from build123d import *

# Parameters (mm, degrees)
ESBO_O1_W                = 90
ESBO_O1_H                = 100
ESBO_O1_W_2              = 13
ESBO_O1_H_2              = 16
RESSALTO_EXTRUS_O1_DEPTH = 2
ESBO_O2_W                = 90
ESBO_O2_H                = 100
ESBO_O2_W_2              = 86
ESBO_O2_H_2              = 96
RESSALTO_EXTRUS_O2_DEPTH = 7


with BuildPart() as part:
    # Esboço1 → Ressalto-extrusão1 (new body)
    with BuildSketch(Plane.XY):
        Rectangle(ESBO_O1_W, ESBO_O1_H)
        with Locations((35.5, 37)):
            Rectangle(ESBO_O1_W_2, ESBO_O1_H_2, mode=Mode.SUBTRACT)
        with Locations((35.5, -37)):
            Rectangle(ESBO_O1_W_2, ESBO_O1_H_2, mode=Mode.SUBTRACT)
        with Locations((-35.5, -37)):
            Rectangle(ESBO_O1_W_2, ESBO_O1_H_2, mode=Mode.SUBTRACT)
        with Locations((-35.5, 37)):
            Rectangle(ESBO_O1_W_2, ESBO_O1_H_2, mode=Mode.SUBTRACT)
    extrude(amount=RESSALTO_EXTRUS_O1_DEPTH)

    # Esboço2 → Ressalto-extrusão2 (add)
    with BuildSketch(Plane.XY.offset(2)):
        Rectangle(ESBO_O2_W, ESBO_O2_H)
        Rectangle(ESBO_O2_W_2, ESBO_O2_H_2, mode=Mode.SUBTRACT)
    extrude(amount=RESSALTO_EXTRUS_O2_DEPTH)


solid = part.part
Source: CAD feature listing. Evaluate the final solid. Frame: model axes, mm. A direction names the side the tool comes from. Round coordinates to 2 decimals unless told otherwise and drop trailing zeros. Order: outer loops, then holes, each group sorted by start corner. A loop starts at its lowest first (then second) coordinate and runs counter-clockwise, first axis right, second up. Notation, with made-up numbers: (5, -17) -> (13, -17) arc R30 cw to (13, 21) -> close; hole circle Ø5 at (-3, 39). An arc over 180 degrees is marked (long way). Answer as CSV lines item,"result".
Item 1: Section B-B, the plane y = 42. Return loops of the section in (x, z).
A:
outline,"(-45, 0) -> (-42, 0) -> (-42, 2) -> (-43, 2) -> (-43, 9) -> (-45, 9) -> close; (-29, 0) -> (29, 0) -> (29, 2) -> (-29, 2) -> close; (42, 0) -> (45, 0) -> (45, 9) -> (43, 9) -> (43, 2) -> (42, 2) -> close"
Item 2: Pull-direction query (Y, two-part tool) for faces 1 (the face through (-45, -1, 4)), 2 (the face through (-1, 50, 4)), 3 (the face through (-1, -50, 4)), 4 (the face through (-1, 1, 2)); classes: pulls with the +Y half, pulls with the -Y half, needs draft (parallel to the pull), parting line crosses it, or undercut.
A:
face 1,"needs draft"
face 2,"pulls with the +Y half"
face 3,"pulls with the -Y half"
face 4,"undercut"
Item 3: Line query: L1, parallel to Y at x = -34, z = 0.5; L2, parallel to X at y = 11.5, z = 7; L3, parallel to Y at x = 3, z = 6.75. Output: solid intervals per line, ascending.
A:
L1,"-50 to -45, -29 to 29, 45 to 50"
L2,"-45 to -43, 43 to 45"
L3,"-50 to -48, 48 to 50"
Item 4: Section C-C, the plane x = 11. Return loops of the section in (y, z), plus the area to 3 significant figures.
A:
outline,"(-50, 0) -> (50, 0) -> (50, 9) -> (48, 9) -> (48, 2) -> (-48, 2) -> (-48, 9) -> (-50, 9) -> close"
area,"228 mm²"
Item 5: Section D-D, the plane y = 7. Return loops of the section in (x, z).
A:
outline,"(-45, 0) -> (45, 0) -> (45, 9) -> (43, 9) -> (43, 2) -> (-43, 2) -> (-43, 9) -> (-45, 9) -> close"
Item 6: Section A-A, the plane z = 3.25. Return loops of the section in (x, y).
A:
outline,"(-45, -50) -> (45, -50) -> (45, 50) -> (-45, 50) -> close; hole (-43, -48) -> (43, -48) -> (43, 48) -> (-43, 48) -> close"
Item 7: Reachability of faces 5 (the face through (-1, 48, 5)), 6 (the face through (45, -1, 4)) from +Z, -Z, +X, -X, +Y, -Y: full face, straight path, thin tool, end or side. Return the list, or none.
A:
face 5,"+Z"
face 6,"+Z, -Z, +X, +Y, -Y"
Item 8: Pin query (flat end, axial travel): pin 1 Ø8 at (x, y) = (-29, -30) entering from +Z. Return the tip coordinate at first contact, or that it passes through.
A:
pin 1,"z = 2"
